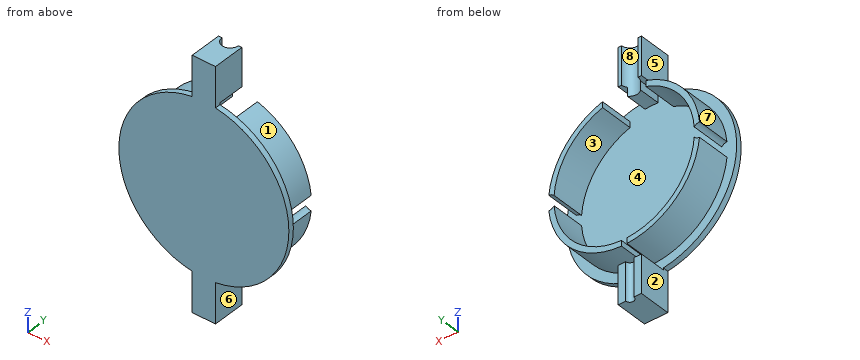
from build123d import *

# Parameters (mm, degrees)
SKETCH1_R                = 31.06
BOSS_EXTRUDE1_DEPTH      = 2
SKETCH2_R                = 27.66
SKETCH2_R_2              = 25.66
BOSS_EXTRUDE2_DEPTH      = 12.25
CUT_EXTRUDE1_DEPTH       = 12.25
CUT_EXTRUDE2_DEPTH       = 6.8
BOSS_EXTRUDE5_DEPTH      = 12.25
CUT_EXTRUDE3_DEPTH       = 7.6
SKETCH9_W                = 2
SKETCH9_H                = 2
SKETCH9_H_2              = 8.25
CUT_EXTRUDE4_DEPTH       = 32.06
CUT_EXTRUDE5_DEPTH       = 12.25
SKETCH12_W               = 4.25
SKETCH12_H               = 14.29
SKETCH12_R               = 31.06
BOSS_EXTRUDE7_DEPTH      = 2
BOSS_EXTRUDE8_DEPTH      = 13.9
BOSS_EXTRUDE9_DEPTH      = 2
BOSS_EXTRUDE9_DEPTH_BACK = 2
BOSS_EXTRUDE10_DEPTH     = 13.9


with BuildPart() as part:
    # Sketch1 → Boss-Extrude1 (new body)
    with BuildSketch(Plane(origin=(0, 0, 0), x_dir=(1, 0, 0), z_dir=(0, 1, 0))):
        Circle(SKETCH1_R)
    extrude(amount=BOSS_EXTRUDE1_DEPTH)

    # Sketch2 → Boss-Extrude2 (add)
    with BuildSketch(Plane(origin=(0, 2, 0), x_dir=(1, 0, 0), z_dir=(0, 1, 0))):
        Circle(SKETCH2_R)
        Circle(SKETCH2_R_2, mode=Mode.SUBTRACT)
    extrude(amount=BOSS_EXTRUDE2_DEPTH)

    # Sketch4 → Cut-Extrude1 (cut)
    with BuildSketch(Plane(origin=(0, 14.25, 0), x_dir=(1, 0, 0), z_dir=(0, 1, 0))):
        with BuildLine():
            ThreePointArc((25.66, 0), (25.643895434, -0.90897027), (25.595601952, -1.816799576))
            ThreePointArc((25.595601952, -1.816799576), (26.465284353, -2.476924408), (27.523295372, -2.746600052))
            ThreePointArc((27.523295372, -2.746600052), (27.625802703, -1.375), (27.66, 0))
            ThreePointArc((27.66, 0), (27.625802703, 1.375), (27.523295372, 2.746600052))
            ThreePointArc((27.523295372, 2.746600052), (26.465284353, 2.476924408), (25.595601952, 1.816799576))
            ThreePointArc((25.595601952, 1.816799576), (25.643895434, 0.90897027), (25.66, 0))
        make_face()
        with BuildLine():
            ThreePointArc((-25.595601952, 1.816799576), (-25.66, 0), (-25.595601952, -1.816799576))
            ThreePointArc((-25.595601952, -1.816799576), (-26.465284353, -2.476924408), (-27.523295372, -2.746600052))
            ThreePointArc((-27.523295372, -2.746600052), (-27.66, 0), (-27.523295372, 2.746600052))
            ThreePointArc((-27.523295372, 2.746600052), (-26.465284353, 2.476924408), (-25.595601952, 1.816799576))
        make_face()
    extrude(amount=-CUT_EXTRUDE1_DEPTH, mode=Mode.SUBTRACT)

    # Sketch5 → Cut-Extrude2 (cut)
    with BuildSketch(Plane(origin=(0, 14.25, 0), x_dir=(1, 0, 0), z_dir=(0, 1, 0))):
        with BuildLine():
            Line((0, -27.66), (0, -25.66))
            ThreePointArc((0, -25.66), (-1.502578344, -25.615968815), (-3, -25.484026369))
            Line((-3, -25.484026369), (-3, -27.496828908))
            ThreePointArc((-3, -27.496828908), (-1.502217095, -27.619177102), (0, -27.66))
        make_face()
        with BuildLine():
            ThreePointArc((3, -25.484026369), (1.502578344, -25.615968815), (0, -25.66))
            Line((0, -25.66), (0, -27.66))
            ThreePointArc((0, -27.66), (1.502217095, -27.619177102), (3, -27.496828908))
            Line((3, -27.496828908), (3, -25.484026369))
        make_face()
    extrude(amount=-CUT_EXTRUDE2_DEPTH, mode=Mode.SUBTRACT)

    # Sketch7 → Boss-Extrude5 (add)
    with BuildSketch(Plane(origin=(0, 2, 0), x_dir=(1, 0, 0), z_dir=(0, 1, 0))):
        with BuildLine():
            Line((2.4, -28.301441659), (2.4, -30.96713742))
            ThreePointArc((2.4, -30.96713742), (0, -31.06), (-2.4, -30.96713742))
            Line((-2.4, -30.96713742), (-2.4, -28.301441659))
            ThreePointArc((-2.4, -28.301441659), (0, -28.402816869), (2.4, -28.301441659))
        make_face()
    extrude(amount=BOSS_EXTRUDE5_DEPTH)

    # Sketch8 → Cut-Extrude3 (cut)
    with BuildSketch(Plane.XY.offset(31.06)):
        with BuildLine():
            ThreePointArc((2.4, 13.55), (2.059119927, 13.931748181), (1.658312395, 14.25))
            Line((1.658312395, 14.25), (-1.658312395, 14.25))
            ThreePointArc((-1.658312395, 14.25), (-2.059119927, 13.931748181), (-2.4, 13.55))
            Line((-2.4, 13.55), (-2.4, 11.75))
            Line((-2.4, 11.75), (2.4, 11.75))
            Line((2.4, 11.75), (2.4, 13.55))
        make_face()
        with BuildLine():
            ThreePointArc((3, 11.75), (2.846049894, 12.698683298), (2.4, 13.55))
            Line((2.4, 13.55), (2.4, 11.75))
            Line((2.4, 11.75), (2.4, 9.95))
            ThreePointArc((2.4, 9.95), (2.846049894, 10.801316702), (3, 11.75))
        make_face()
        with BuildLine():
            Line((2.4, 9.95), (2.4, 11.75))
            Line((2.4, 11.75), (-2.4, 11.75))
            Line((-2.4, 11.75), (-2.4, 9.95))
            ThreePointArc((-2.4, 9.95), (0, 8.75), (2.4, 9.95))
        make_face()
        with BuildLine():
            Line((-2.4, 11.75), (-2.4, 13.55))
            ThreePointArc((-2.4, 13.55), (-3, 11.75), (-2.4, 9.95))
            Line((-2.4, 9.95), (-2.4, 11.75))
        make_face()
        with BuildLine():
            Line((2.4, 13.55), (2.4, 14.25))
            Line((2.4, 14.25), (1.658312395, 14.25))
            ThreePointArc((1.658312395, 14.25), (2.059119927, 13.931748181), (2.4, 13.55))
        make_face()
        with BuildLine():
            ThreePointArc((-2.4, 13.55), (-2.059119927, 13.931748181), (-1.658312395, 14.25))
            Line((-1.658312395, 14.25), (-2.4, 14.25))
            Line((-2.4, 14.25), (-2.4, 13.55))
        make_face()
    extrude(amount=-CUT_EXTRUDE3_DEPTH, mode=Mode.SUBTRACT)

    # Sketch9 → Cut-Extrude4 (cut, through all)
    with BuildSketch(Plane.XY):
        with Locations((0, 5)):
            Rectangle(SKETCH9_W, SKETCH9_H)
        with Locations((0, 10.125)):
            Rectangle(SKETCH9_W, SKETCH9_H_2)
    extrude(amount=-CUT_EXTRUDE4_DEPTH, mode=Mode.SUBTRACT)

    # Sketch11 → Cut-Extrude5 (cut)
    with BuildSketch(Plane(origin=(0, 14.25, 0), x_dir=(1, 0, 0), z_dir=(0, 1, 0))):
        with BuildLine():
            ThreePointArc((3, -27.496828908), (5.472387467, -27.113254607), (7.9, -26.50784035))
            Line((7.9, -26.50784035), (7.9, -24.413635534))
            ThreePointArc((7.9, -24.413635534), (5.476215311, -25.068838542), (3, -25.484026369))
            Line((3, -25.484026369), (3, -27.496828908))
        make_face()
        with BuildLine():
            Line((-7.9, -26.50784035), (-7.9, -27.987377494))
            Line((-7.9, -27.987377494), (7.9, -27.987377494))
            Line((7.9, -27.987377494), (7.9, -26.50784035))
            ThreePointArc((7.9, -26.50784035), (5.472387467, -27.113254607), (3, -27.496828908))
            Line((3, -27.496828908), (3, -25.484026369))
            ThreePointArc((3, -25.484026369), (5.476215311, -25.068838542), (7.9, -24.413635534))
            Line((7.9, -24.413635534), (7.9, -24.165769621))
            Line((7.9, -24.165769621), (-7.9, -24.165769621))
            Line((-7.9, -24.165769621), (-7.9, -24.413635534))
            ThreePointArc((-7.9, -24.413635534), (-5.476215311, -25.068838542), (-3, -25.484026369))
            Line((-3, -25.484026369), (-3, -27.496828908))
            ThreePointArc((-3, -27.496828908), (-5.472387467, -27.113254607), (-7.9, -26.50784035))
        make_face()
        with BuildLine():
            Line((-7.9, -24.413635534), (-7.9, -26.50784035))
            ThreePointArc((-7.9, -26.50784035), (-5.472387467, -27.113254607), (-3, -27.496828908))
            Line((-3, -27.496828908), (-3, -25.484026369))
            ThreePointArc((-3, -25.484026369), (-5.476215311, -25.068838542), (-7.9, -24.413635534))
        make_face()
    extrude(amount=-CUT_EXTRUDE5_DEPTH, mode=Mode.SUBTRACT)

    # Sketch12 → Boss-Extrude7 (add)
    with BuildSketch(Plane.XZ):
        with Locations((2.125, 38.205)):
            Rectangle(SKETCH12_W, SKETCH12_H)
        with Locations((-2.125, 38.205)):
            Rectangle(SKETCH12_W, SKETCH12_H)
        with BuildLine():
            Line((4.25, 31.06), (0, 31.06))
            ThreePointArc((0, 31.06), (2.130014484, 30.986878486), (4.25, 30.767858229))
            Line((4.25, 30.767858229), (4.25, 31.06))
        make_face()
        with BuildLine():
            ThreePointArc((-4.25, 30.767858229), (-2.130014484, 30.986878486), (0, 31.06))
            Line((0, 31.06), (-4.25, 31.06))
            Line((-4.25, 31.06), (-4.25, 30.767858229))
        make_face()
        with Locations((2.125, -38.205)):
            Rectangle(SKETCH12_W, SKETCH12_H)
        with Locations((-2.125, -38.205)):
            Rectangle(SKETCH12_W, SKETCH12_H)
        with BuildLine():
            ThreePointArc((0, -31.06), (-2.130014484, -30.986878486), (-4.25, -30.767858229))
            Line((-4.25, -30.767858229), (-4.25, -31.06))
            Line((-4.25, -31.06), (0, -31.06))
        make_face()
        with BuildLine():
            Line((4.25, -31.06), (4.25, -30.767858229))
            ThreePointArc((4.25, -30.767858229), (2.130014484, -30.986878486), (0, -31.06))
            Line((0, -31.06), (4.25, -31.06))
        make_face()
        Circle(SKETCH12_R)
    extrude(amount=-BOSS_EXTRUDE7_DEPTH)

    # Sketch13 → Boss-Extrude8 (add)
    with BuildSketch(Plane.XY.offset(45.35)):
        with BuildLine():
            Line((-3, 11.75), (-4.25, 11.75))
            Line((-4.25, 11.75), (-4.25, 2))
            Line((-4.25, 2), (4.25, 2))
            Line((4.25, 2), (4.25, 11.75))
            Line((4.25, 11.75), (3, 11.75))
            ThreePointArc((3, 11.75), (0, 8.75), (-3, 11.75))
        make_face()
    extrude(amount=-BOSS_EXTRUDE8_DEPTH)

    # Sketch14 → Boss-Extrude9 (add, two sides)
    with BuildSketch(Plane.XY.offset(31.06)) as boss_extrude9_sk:
        with BuildLine():
            Line((-2.4, 2), (2.4, 2))
            Line((2.4, 2), (2.4, 9.95))
            ThreePointArc((2.4, 9.95), (0, 8.75), (-2.4, 9.95))
            Line((-2.4, 9.95), (-2.4, 2))
        make_face()
    extrude(amount=BOSS_EXTRUDE9_DEPTH)
    extrude(boss_extrude9_sk.sketch, amount=-BOSS_EXTRUDE9_DEPTH_BACK)

    # Sketch15 → Boss-Extrude10 (add)
    with BuildSketch(Plane(origin=(0, 0, -45.35), x_dir=(-1, 0, 0), z_dir=(0, 0, -1))):
        with BuildLine():
            Line((-1.5, 11.75), (-4.25, 11.75))
            Line((-4.25, 11.75), (-4.25, 0))
            Line((-4.25, 0), (4.25, 0))
            Line((4.25, 0), (4.25, 11.75))
            Line((4.25, 11.75), (1.5, 11.75))
            ThreePointArc((1.5, 11.75), (0, 10.25), (-1.5, 11.75))
        make_face()
    extrude(amount=-BOSS_EXTRUDE10_DEPTH)


solid = part.part
Geometry check sheet. Reference: the model listing, model coordinates, mm. Face numbers are marked on the shaded views. A direction names the side the tool comes from. Give positions to 0.01 mm unless a question says otherwise; leave off trailing zeros. Order: outer loops, then holes, each group sorted by start corner. A loop starts at its lowest first (then second) coordinate and runs counter-clockwise, first axis right, second up.
1) Cross-section at A-A (y = 5.5). Record the boundary of the cut face in (x, z), then the cut area to 3 significant figures.
Results are:
outline: (-27.52, -2.75) arc R27.66 ccw to (-1, -27.64) - (-1, -25.64) arc R25.66 cw to (-25.6, -1.82) arc R2.75 cw to start; (-27.52, 2.75) arc R2.75 cw to (-25.6, 1.82) arc R25.66 cw to (-7.9, 24.41) - (-7.9, 26.51) arc R27.66 ccw to start; (-4.25, -45.35) - (4.25, -45.35) - (4.25, -31.45) - (-4.25, -31.45) - close; (-4.25, 31.45) - (-2.4, 31.45) - (-2.4, 28.3) arc R28.46 cw to (2.4, 28.3) - (2.4, 31.45) - (4.25, 31.45) - (4.25, 45.35) - (-4.25, 45.35) - close; (1, -27.64) arc R27.66 ccw to (27.52, -2.75) arc R2.75 cw to (25.6, -1.82) arc R25.66 cw to (1, -25.64) - close; (7.9, 24.41) arc R25.66 cw to (25.6, 1.82) arc R2.75 cw to (27.52, 2.75) arc R27.66 ccw to (7.9, 26.51) - close
area: 530 mm2
2) Tool access check on the marked faces 5, 6, 7 and 8. Record the directions out of +Z, -Z, +X, -X, +Y, -Y that give a thin tool (end or side, any length) a straight path to the whole face; none if there is none.
Results are:
face 5: +Z, -X, +Y, -Y
face 6: -Z, +X, +Y, -Y
face 7: +Z, -X, +Y
face 8: +Z, +Y
3) Cross-section at C-C (z = -23). Record the boundary of the cut face in (x, y).
Results are:
outline: (-20.87, 0) - (20.87, 0) - (20.87, 2) - (15.36, 2) - (15.36, 14.25) - (11.38, 14.25) - (11.38, 2) - (-11.38, 2) - (-11.38, 14.25) - (-15.36, 14.25) - (-15.36, 2) - (-20.87, 2) - close
4) Material ranges on probe 1 along Z at (x, y) = (1.5, 7.25); probe 2 along Z at (x, y) = (2, 7); probe 3 along X at (y, z) = (3.75, 29.5), recorded low to high.
Results are:
probe 1: z = -45.35 to -31.45, -27.62 to -25.62, 28.36 to 45.35
probe 2: z = -45.35 to -31.45, -27.59 to -25.58, 28.33 to 45.35
probe 3: x = -2.4 to 2.4
5) Cross-section at B-B (x = 0). Record the boundary of the cut face in (y, z).
Results are:
outline: (0, -45.35) - (10.25, -45.35) - (10.25, -31.45) - (2, -31.45) - (2, -27.66) - (4, -27.66) - (4, -25.66) - (2, -25.66) - (2, 28.4) - (8.75, 28.4) - (8.75, 45.35) - (0, 45.35) - close
6) Gauge pin test, flat ends, axial feed: pin 1 (1 mm diameter, centred on x = 24.5, y = 11, fed in from -Z); pin 2 (1.4 mm diameter, centred on x = 3.5, z = 35.5, fed in from +Y); pin 3 (1 mm diameter, centred on x = 0, z = -27, fed in from +Y). Record the tip position at first contact, or that the pin passes through.
Results are:
pin 1: stops at z = -13.75
pin 2: stops at y = 11.75
pin 3: stops at y = 4
7) Draft check along X on the marked faces 1, 2, 3 and 4. Enter one of: released by +X, released by -X, zero draft, split by the parting line, or undercut.
Results are:
face 1: released by +X
face 2: released by -X
face 3: undercut
face 4: undercut
